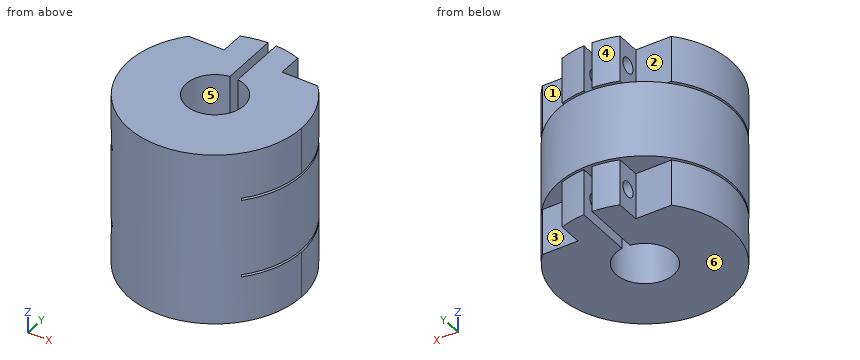
Autodesk Inventor part; units mm, degrees
ref_plane "Work Plane1" through (0, 0, 9.525) normal (0, 0, -1) x (-1, 0, 0)
ref_plane "YZ Plane" through (0, 0, 0) normal (1, 0, 0) x (0, 1, 0)
ref_plane "XZ Plane" through (0, 0, 0) normal (0, 1, 0) x (-1, 0, 0)
sketch "Sketch1" plane through (0, 0, 0) normal (0, 0, 1) x (1, 0, 0)
  circle A0 centre (0, 0) radius 9.525
  circle A1 centre (0, 0) radius 3.175
  line L0 (0, 0) -> (-0.4464, 0)
  line L1 (-0.4464, 0) -> (-0.4464, 9.5145)
  line L2 (0, 0) -> (0.4464, 0)
  line L3 (0.4464, 0) -> (0.4464, 9.5145)
  line L4 (0, 0) -> (0, 9.525)
  line L5 (-7.0995, 6.35) -> (-3.175, 6.35)
  line L6 (-3.175, 6.35) -> (-3.175, 8.9803)
  line L7 (3.175, 8.9803) -> (3.175, 6.35)
  line L8 (3.175, 6.35) -> (7.0995, 6.35)
  dimension "d0" = 19.05
  dimension "d1" = 6.35
  dimension "d4" = 3.175
  dimension "d5" = 0.4464
  dimension "d6" = 3.175
  dimension "d7" = 3.175
extrude "Extrusion1" add sketch "Sketch1" along normal blind 19.05
extrude "Extrusion2" cut sketch "Sketch1" along normal blind 5.334 contours L8 L7 A0 | A0 L6 L5 | L3 A1 L4 A0 | A0 L4 A1 L1 | L3 L2 L4 A1 | A1 L1 L0 L2 L3 | A1 L4 L0 L1
sketch "Sketch2" plane through (0, 0, 5.334) normal (0, 0, -1) x (-1, 0, 0)
  line L0 (-3.175, 8.9803) -> (-3.175, 6.35)
  arc A0 (-3.175, 8.9803) -> (-7.0995, 6.35) centre (0, 0) ccw
  line L1 (-3.175, 6.35) -> (-7.0995, 6.35)
  circle A1 centre (0, 0) radius 9.525
  line L2 (-7.0995, -6.35) -> (7.0995, -6.35)
  dimension "d10" = 6.35
extrude "Extrusion3" cut sketch "Sketch2" along normal blind 0.254 contours A1 L2 L1 L0
ref_plane "Work Plane1" through (0, 0, 9.525) normal (0, 0, -1) x (-1, 0, 0)
sketch "Sketch3" plane through (3.175, 6.35, 0) normal (1, 0, 0) x (0, 0, -1)
  line L0 (0, 0) -> (-5.08, 0)
  line L1 (0, 2.6303) -> (0, 0)
  point P0 (0, -6.35)
  point P1 (-2.54, 1.3151)
  dimension "d14" = 2.54
  dimension "d15" = 1.3151
hole "Hole1" at (3.175, 7.6651, 2.54) direction (-1, 0, 0) diameter 1.7018 depth 25.4 tip angle 118
mirror "Mirror1" about plane through (0, 0, 9.525) normal (0, 0, -1) of "Extrusion2", "Extrusion3", "Hole1"
equation "\"d7\" = d6"
properties part number "Flexible Shaft Coupler 6208K411"
Can you work these out from the model? Positions are in its coordinate system, mm. Face numbers are marked on the shaded views. A direction names the side the tool comes from. Give positions to 0.01 mm unless a question says otherwise; leave off trailing zeros. Loops run counter-clockwise (first coordinate to the right, second up) from the corner with the lowest first, then second, coordinate; pieces in that order, holes last. Notation, with made-up numbers: M 36,29 L 59,29 A18 cw 59,36 Z; hole C -27,65.5 d4. An arc over 180 degrees is marked long. One line per item, written item: value.
(1) Will these pins go through, and if not, where does the flat tip stop? pin 1 (6 mm diameter, centred on y = -6, z = 2, fed in from -X); pin 2 (1 mm diameter, centred on x = 2, z = 10.5, fed in from +Y); pin 3 (4 mm diameter, centred on x = -1.5, y = -2, fed in from +Z); pin 4 (4.5 mm diameter, centred on x = -6, z = 2, fed in from +Y).
Returned:
pin 1: x = -9.04
pin 2: y = 9.41
pin 3: z = 19.05
pin 4: y = 6.35
(2) Suppose I cut it at B-B on z = 16.51. Count the separate pieces of the cut face and the enclosed holes in it, plus the area to 3 significant figures.
Returned:
separate pieces: 3
enclosed holes: 0
area: 226 mm^2
(3) We'd pull the mould along X, two halves only. Please class the marked faces 4, 5 and 6: released by +X, released by -X, zero draft, split by the parting line, or undercut.
Returned:
face 4: released by -X
face 5: undercut
face 6: zero draft
(4) Suppose I cut it at A-A on x = 0. List the corners of the cut face in (y, z) for me (3 decimals), plus the area to 3 significant figures.
Returned:
outline: M -9.525,0 L -3.175,0 L -3.175,5.08 L -6.35,5.08 L -6.35,5.334 L 9.525,5.334 L 9.525,13.716 L -6.35,13.716 L -6.35,13.97 L -3.175,13.97 L -3.175,19.05 L -9.525,19.05 Z
area: 226 mm^2
(5) Suppose I cut it at D-D on z = 10.75. List the corners of the cut face in (x, y) for me (3 decimals).
Returned:
outline: C 0,0 d19.05
(6) I need wall thicknesses on line 1 (Z direction, x = -2, y = -3.25); line 2 (X direction, y = 0, z = 3.5) (3 decimals); line 3 (Y direction, x = -2.25, z = 16.51). Which ranges of each line are inside material? Lowest first, please.
Returned:
line 1: 0 to 5.08, 5.33 to 13.72, 13.97 to 19.05
line 2: -9.525 to -3.175, 3.175 to 9.525
line 3: -9.26 to -2.24, 2.24 to 6.81, 8.52 to 9.26
(7) Which directions (+Z, -Z, +X, -X, +Y, -Y) give clear straight access to the entire face, cutting with the end or side of a thin tool? Please do the marked faces 1, 2 and 3.
Returned:
face 1: +Z, +X, +Y
face 2: +Z, -X, +Y
face 3: -Z, +X, +Y
(8) Suppose I cut it at C-C on y = 4.5. List the corners of the cut face in (x, z) for me, plus the area to 3 significant figures.
Returned:
outline: M -8.39,0 L -0.45,0 L -0.45,5.08 L -8.39,5.08 Z; M -8.39,5.33 L 8.39,5.33 L 8.39,13.72 L -8.39,13.72 Z; M -8.39,13.97 L -0.45,13.97 L -0.45,19.05 L -8.39,19.05 Z; M 0.45,0 L 8.39,0 L 8.39,5.08 L 0.45,5.08 Z; M 0.45,13.97 L 8.39,13.97 L 8.39,19.05 L 0.45,19.05 Z
area: 302 mm^2
